Could you check a few things on this model? Use its own coordinates, in mm. Face numbers are marked on the shaded views. A direction names the side the tool comes from. Coordinates: 2 decimals unless noted, no trailing zeros. Loops run counter-clockwise (first coordinate to the right, second up) from the corner with the lowest first, then second, coordinate; pieces in that order, holes last.
1) If I drill on line 1 along Y through (x, z) = (33, -2.5); line 2 along Z through (x, y) = (30, 114.5); line 3 along Y through (x, z) = (11, -12), over which ranges is the centre line in solid material (lowest first)?
2) Imagine slicing it at C-C on x = 3.5. Please give me the cut outline in (y, z), plus the area to 3 significant figures.
3) Imagine slicing it at D-D on x = 37. Please give me the cut outline in (y, z), plus the area to 3 significant figures.
4) Imagine slicing it at A-A on z = -5. Please give me the cut outline in (x, y) (3 decimals).
5) Will these pins go through, and if not, where does the flat tip stop? P1, Ø5, axis at x = 36, y = 96, coming from the -Z side; P2, Ø2, axis at x = 32.5, y = 31.5, coming from the -Z side; P3, Ø3.5, axis at x = 41, z = -5, coming from the +Y side.
6) Imagine slicing it at B-B on y = 63.5. Please give me the cut outline in (x, z), plus the area to 3 significant figures.
7) Thinking about a two-plate mould opening in Y: for the marked faces 5, 6, 7 and 8, which applies, released by +Y, released by -Y, zero draft, split by the parting line, or undercut?
8) For the marked faces 1, 2, 3 and 4, which set-ups out of +Z, -Z, +X, -X, +Y, -Y let a thin tool reach every point of the face, with its end or its side?
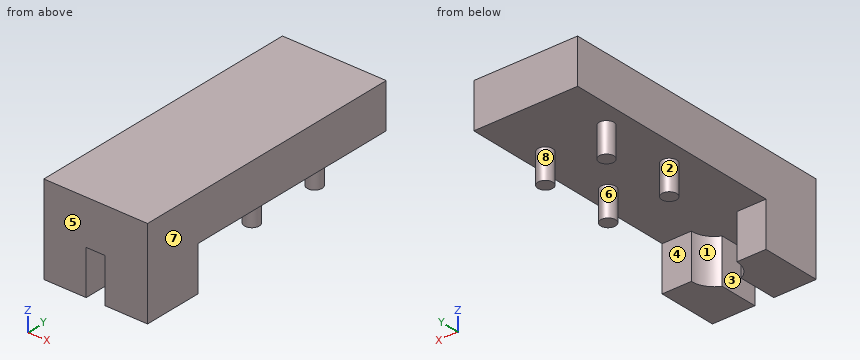
```python
from build123d import *

# Parameters (mm, degrees)
SKETCH1_W           = 44.45
SKETCH1_H           = 120.65
BOSS_EXTRUDE1_DEPTH = 19.05
BOSS_EXTRUDE2_DEPTH = 19.05
SKETCH2_4_R         = 3.175
BOSS_EXTRUDE3_DEPTH = 12.7


with BuildPart() as part:
    # Sketch1 → Boss-Extrude1 (new body)
    with BuildSketch(Plane.XY):
        with Locations((22.225, 60.325)):
            Rectangle(SKETCH1_W, SKETCH1_H)
    extrude(amount=BOSS_EXTRUDE1_DEPTH)

    # Sketch2 → Boss-Extrude2 (add)
    with BuildSketch(Plane(origin=(0, 0, 0), x_dir=(-1, 0, 0), z_dir=(0, 0, -1))):
        with BuildLine():
            ThreePointArc((-26.281784125, 16.521928603), (-30.437065172, 20.123672226), (-31.986027055, 25.4))
            Line((-31.986027055, 25.4), (-44.45, 25.4))
            Line((-44.45, 25.4), (-44.45, 0))
            Line((-44.45, 0), (-26.281784125, 0))
            Line((-26.281784125, 0), (-26.281784125, 16.521928603))
        make_face()
        with BuildLine():
            Line((0, 25.4), (-12.463972945, 25.4))
            ThreePointArc((-12.463972945, 25.4), (-14.012934828, 20.123672226), (-18.168215875, 16.521928603))
            Line((-18.168215875, 16.521928603), (-18.168215875, 0))
            Line((-18.168215875, 0), (0, 0))
            Line((0, 0), (0, 25.4))
        make_face()
    extrude(amount=BOSS_EXTRUDE2_DEPTH)

    # Sketch2_4 → Boss-Extrude3 (add)
    with BuildSketch(Plane(origin=(0, 0, 0), x_dir=(-1, 0, 0), z_dir=(0, 0, -1))):
        with Locations((-35.306, 95.25)):
            Circle(SKETCH2_4_R)
        with Locations((-35.306, 63.5)):
            Circle(SKETCH2_4_R)
        with Locations((-9.144, 95.25)):
            Circle(SKETCH2_4_R)
        with Locations((-9.144, 63.5)):
            Circle(SKETCH2_4_R)
    extrude(amount=BOSS_EXTRUDE3_DEPTH)


solid = part.part
```
Filled in:
1. line 1: y = 0 to 25.4, 61.32 to 65.68, 93.07 to 97.43
1. line 2: z = 0 to 19.05
1. line 3: y = 0 to 25.4, 60.92 to 66.08, 92.67 to 97.83
2. outline: (0, -19.05) - (25.4, -19.05) - (25.4, 0) - (120.65, 0) - (120.65, 19.05) - (0, 19.05) - close
2. area: 2,780 mm2
3. outline: (0, -19.05) - (25.4, -19.05) - (25.4, 0) - (60.81, 0) - (60.81, -12.7) - (66.19, -12.7) - (66.19, 0) - (92.56, 0) - (92.56, -12.7) - (97.94, -12.7) - (97.94, 0) - (120.65, 0) - (120.65, 19.05) - (0, 19.05) - close
3. area: 2,920 mm2
4. outline: (0, 0) - (18.168, 0) - (18.168, 16.522) arc R9.761 cw to (12.464, 25.4) - (0, 25.4) - close; circle Ø6.35 at (9.144, 63.5); circle Ø6.35 at (9.144, 95.25); (26.282, 0) - (44.45, 0) - (44.45, 25.4) - (31.986, 25.4) arc R9.761 cw to (26.282, 16.522) - close; circle Ø6.35 at (35.306, 63.5); circle Ø6.35 at (35.306, 95.25)
5. P1: stops at z = -12.7
5. P2: stops at z = 0
5. P3: stops at y = 25.4
6. outline: (0, 0) - (5.97, 0) - (5.97, -12.7) - (12.32, -12.7) - (12.32, 0) - (32.13, 0) - (32.13, -12.7) - (38.48, -12.7) - (38.48, 0) - (44.45, 0) - (44.45, 19.05) - (0, 19.05) - close
6. area: 1,010 mm2
7. face 5: released by -Y
7. face 6: undercut
7. face 7: zero draft
7. face 8: undercut
8. face 1: -Z, +Y
8. face 2: -Z
8. face 3: -Z, +Y, -Y
8. face 4: -Z, +X, -X
